```python
from build123d import *

# Parameters (mm, degrees)
SKETCH1_R           = 2.25
SKETCH1_R_2         = 1.6
SKETCH1_W           = 3
SKETCH1_H           = 10
BOSS_EXTRUDE1_DEPTH = 3
SKETCH2_R           = 0.5
CUT_EXTRUDE1_DEPTH  = 4


with BuildPart() as part:
    # Sketch1 → Boss-Extrude1 (new body)
    with BuildSketch(Plane(origin=(0, 0, 0), x_dir=(1, 0, 0), z_dir=(0, 1, 0))):
        with BuildLine():
            Line((-46, -20), (46, -20))
            ThreePointArc((46, -20), (47.414213562, -19.414213562), (48, -18))
            Line((48, -18), (48, 18))
            ThreePointArc((48, 18), (47.414213562, 19.414213562), (46, 20))
            Line((46, 20), (-46, 20))
            ThreePointArc((-46, 20), (-47.414213562, 19.414213562), (-48, 18))
            Line((-48, 18), (-48, -18))
            ThreePointArc((-48, -18), (-47.414213562, -19.414213562), (-46, -20))
        make_face()
        with Locations((-30, 13.1)):
            Circle(SKETCH1_R, mode=Mode.SUBTRACT)
        with Locations((30, 13.1)):
            Circle(SKETCH1_R, mode=Mode.SUBTRACT)
        with Locations((30, -13.1)):
            Circle(SKETCH1_R, mode=Mode.SUBTRACT)
        with Locations((-30, -13.1)):
            Circle(SKETCH1_R, mode=Mode.SUBTRACT)
        with Locations((41.5, 0)):
            Circle(SKETCH1_R_2, mode=Mode.SUBTRACT)
        with Locations((-41.5, 0)):
            Circle(SKETCH1_R_2, mode=Mode.SUBTRACT)
        with Locations((-41.5, 10)):
            Rectangle(SKETCH1_W, SKETCH1_H, mode=Mode.SUBTRACT)
        with Locations((-41.5, -10)):
            Rectangle(SKETCH1_W, SKETCH1_H, mode=Mode.SUBTRACT)
        with Locations((41.5, 10)):
            Rectangle(SKETCH1_W, SKETCH1_H, mode=Mode.SUBTRACT)
        with Locations((41.5, -10)):
            Rectangle(SKETCH1_W, SKETCH1_H, mode=Mode.SUBTRACT)
    extrude(amount=BOSS_EXTRUDE1_DEPTH)

    # Sketch2 → Cut-Extrude1 (cut, through all)
    with BuildSketch(Plane(origin=(0, 3, 0), x_dir=(1, 0, 0), z_dir=(0, 1, 0))):
        with Locations((-43, 15)):
            Circle(SKETCH2_R)
        with Locations((-40, 15)):
            Circle(SKETCH2_R)
        with Locations((-40, 5)):
            Circle(SKETCH2_R)
        with Locations((-43, 5)):
            Circle(SKETCH2_R)
        with Locations((-43, -5)):
            Circle(SKETCH2_R)
        with Locations((-40, -5)):
            Circle(SKETCH2_R)
        with Locations((-43, -15)):
            Circle(SKETCH2_R)
        with Locations((-40, -15)):
            Circle(SKETCH2_R)
        with Locations((40, -15)):
            Circle(SKETCH2_R)
        with Locations((43, -15)):
            Circle(SKETCH2_R)
        with Locations((43, -5)):
            Circle(SKETCH2_R)
        with Locations((40, -5)):
            Circle(SKETCH2_R)
        with Locations((40, 5)):
            Circle(SKETCH2_R)
        with Locations((43, 5)):
            Circle(SKETCH2_R)
        with Locations((43, 15)):
            Circle(SKETCH2_R)
        with Locations((40, 15)):
            Circle(SKETCH2_R)
    extrude(amount=-CUT_EXTRUDE1_DEPTH, mode=Mode.SUBTRACT)


solid = part.part
```
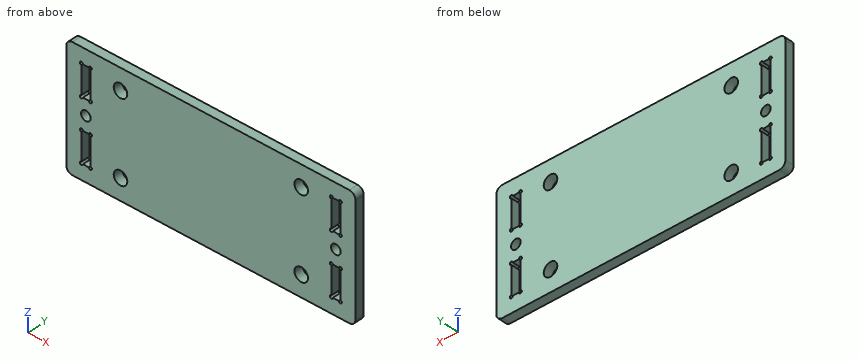
Build history of the part. All positions in model axes, mm. Round coordinates to 2 decimals unless told otherwise and drop trailing zeros. Loops run counter-clockwise (first coordinate to the right, second up) from the corner with the lowest first, then second, coordinate; pieces in that order, holes last.
Item 1: Saw through at A-A (z = 0). List the corners of the cut face in (x, y).
Item 2: Saw through at B-B (x = 41.5). List the corners of the cut face in (y, z), then the cut area to 3 significant figures.
Item 3: Drill centre lines: line 1 along X through (y, z) = (1.55, -13.1); line 2 along X through (y, z) = (0.6, 0.5); line 3 along Z through (x, y) = (41.5, 2.15). Where is each one in solid material? Low to high.
Item 4: Saw through at C-C (x = -30). List the corners of the cut face in (y, z), then the cut area to 3 significant figures.
Item 5: Saw through at D-D (y = 2.5). State how many separate pieces and enclosed holes the cut face has, then the cut area to 3 significant figures.
Worked answers:
1. outline: (-48, 0) - (-43.1, 0) - (-43.1, 3) - (-48, 3) - close; (-39.9, 0) - (39.9, 0) - (39.9, 3) - (-39.9, 3) - close; (43.1, 0) - (48, 0) - (48, 3) - (43.1, 3) - close
2. outline: (0, -20) - (3, -20) - (3, -15) - (0, -15) - close; (0, -5) - (3, -5) - (3, -1.6) - (0, -1.6) - close; (0, 1.6) - (3, 1.6) - (3, 5) - (0, 5) - close; (0, 15) - (3, 15) - (3, 20) - (0, 20) - close
2. area: 50.4 mm2
3. line 1: x = -48 to -43, -40 to -32.25, -27.75 to 27.75, 32.25 to 40, 43 to 48
3. line 2: x = -48 to -43.02, -39.98 to 39.98, 43.02 to 48
3. line 3: z = -20 to -15, -5 to -1.6, 1.6 to 5, 15 to 20
4. outline: (0, -20) - (3, -20) - (3, -15.35) - (0, -15.35) - close; (0, -10.85) - (3, -10.85) - (3, 10.85) - (0, 10.85) - close; (0, 15.35) - (3, 15.35) - (3, 20) - (0, 20) - close
4. area: 93.0 mm2
5. separate pieces: 1
5. enclosed holes: 10
5. area: 3,630 mm2
